Could you check a few things on this model? Use its own coordinates, in mm. Round coordinates to 2 decimals unless told otherwise and drop trailing zeros. Loops run counter-clockwise (first coordinate to the right, second up) from the corner with the lowest first, then second, coordinate; pieces in that order, holes last. Notation, with made-up numbers: (84, 28) -> (103, 28) arc R26 cw to (103, 55) -> close; hole circle Ø11 at (3, 8.5). An arc over 180 degrees is marked (long way). Write each question's results on one line, items separated by ' | '.
from build123d import *

# Parameters (mm, degrees)
F1_DEPTH = 50


with BuildPart() as f1:
    # F0 (on Front) → F1 (new body)
    with BuildSketch(Plane.XZ):
        with BuildLine():
            Line((91.4418067738, 17.4405043857), (4.1054428346, 24.6606029758))
            ThreePointArc((4.1054428346, 24.6606029758), (19.0740146648, 16.1611251022), (25, 0))
            ThreePointArc((25, 0), (19.0740146648, -16.1611251022), (4.1054428346, -24.6606029758))
            Line((4.1054428346, -24.6606029758), (91.4418067738, -17.4405043857))
            ThreePointArc((91.4418067738, -17.4405043857), (72.5, 0), (91.4418067738, 17.4405043857))
        make_face()
        with BuildLine():
            Line((4.1054428346, 24.6606029758), (0, 25))
            ThreePointArc((0, 25), (-25, 0), (0, -25))
            Line((0, -25), (4.1054428346, -24.6606029758))
            ThreePointArc((4.1054428346, -24.6606029758), (19.0740146648, -16.1611251022), (25, 0))
            ThreePointArc((25, 0), (19.0740146648, 16.1611251022), (4.1054428346, 24.6606029758))
        make_face()
        with BuildLine():
            ThreePointArc((107.5, 0), (102.8740362463, 11.8536572723), (91.4418067738, 17.4405043857))
            ThreePointArc((91.4418067738, 17.4405043857), (72.5, 0), (91.4418067738, -17.4405043857))
            ThreePointArc((91.4418067738, -17.4405043857), (102.8740362463, -11.8536572723), (107.5, 0))
        make_face()
    extrude(amount=F1_DEPTH)


solid = f1.part
1) I need wall thicknesses on line 1 (Z direction, x = -4, y = -3); line 2 (X direction, y = -17, z = -13.5); line 3 (Z direction, x = 46, y = -11.5). Which ranges of each line are inside material? Lowest first, please.
Model answer:
line 1: z = -24.68 to 24.68 | line 2: x = -21.04 to 101.14 | line 3: z = -21.2 to 21.2
2) I want a section at C-C, the plane x = 34. Write out the boundary of the cut face in (y, z).
Model answer:
outline: (-50, -22.19) -> (0, -22.19) -> (0, 22.19) -> (-50, 22.19) -> close
3) I'm going to push flat-ended pins straight in: pin 1 (6 mm diameter, centred on x = 69.5, y = -14, fed in from +Z); pin 2 (1 mm diameter, centred on x = 58.5, y = -13, fed in from -Z); pin 3 (12 mm diameter, centred on x = 84, y = -40, fed in from +Z). Where does each tip first touch, or does it pass through?
Model answer:
pin 1: stops at z = 19.5 | pin 2: stops at z = -20.21 | pin 3: stops at z = 18.55
4) I want a section at B-B, the plane z = -10.5. Write out the boundary of the cut face in (x, y), plus the area to 3 significant figures.
Model answer:
outline: (-22.69, -50) -> (104, -50) -> (104, 0) -> (-22.69, 0) -> close | area: 6,330 mm2
5) I want a section at A-A, the plane y = -14. Write out the boundary of the cut face in (x, z).
Model answer:
outline: (0, -25) -> (91.44, -17.44) arc R17.5 ccw to (91.44, 17.44) -> (0, 25) arc R25 ccw to start
